Verification items for this drawing (mm, ordinates from the low corner). Round coordinates to 2 decimals unless told otherwise and drop trailing zeros. Order: outer loops, then holes, each group sorted by start corner. A loop starts at its lowest first (then second) coordinate and runs counter-clockwise, first axis right, second up. Notation, with made-up numbers: M -38.5,4.5 L -4.5,4.5 A20 cw -4.5,31.5 Z; hole C 1.25,85 d1. An arc over 180 degrees is marked long. One line per item, written item: value. Start each with the question number.
(1) Cross-section at A-A, the plane x = 3. Enter the section's corners in (y, z).
(2) Cross-section at C-C, the plane y = 1.1. Enter the section's corners in (x, z), and give its area (3 significant figures).
(3) Cross-section at D-D, the plane z = 9. Enter the section's corners in (x, y).
(4) Release check for a two-part mould opening along X. For the marked faces 1, 2 and 3 record: released by +X, released by -X, zero draft, split by the parting line, or undercut.
(5) Cross-section at B-B, the plane x = 11. Enter the section's corners in (y, z).
(6) Thickness scan on L1, parallel to Z at x = 3, y = 1.15; L2, parallel to X at y = 1, z = 7.5; L3, parallel to X at y = 0.65, z = 5.75. Record the ranges inside material, lowest first.
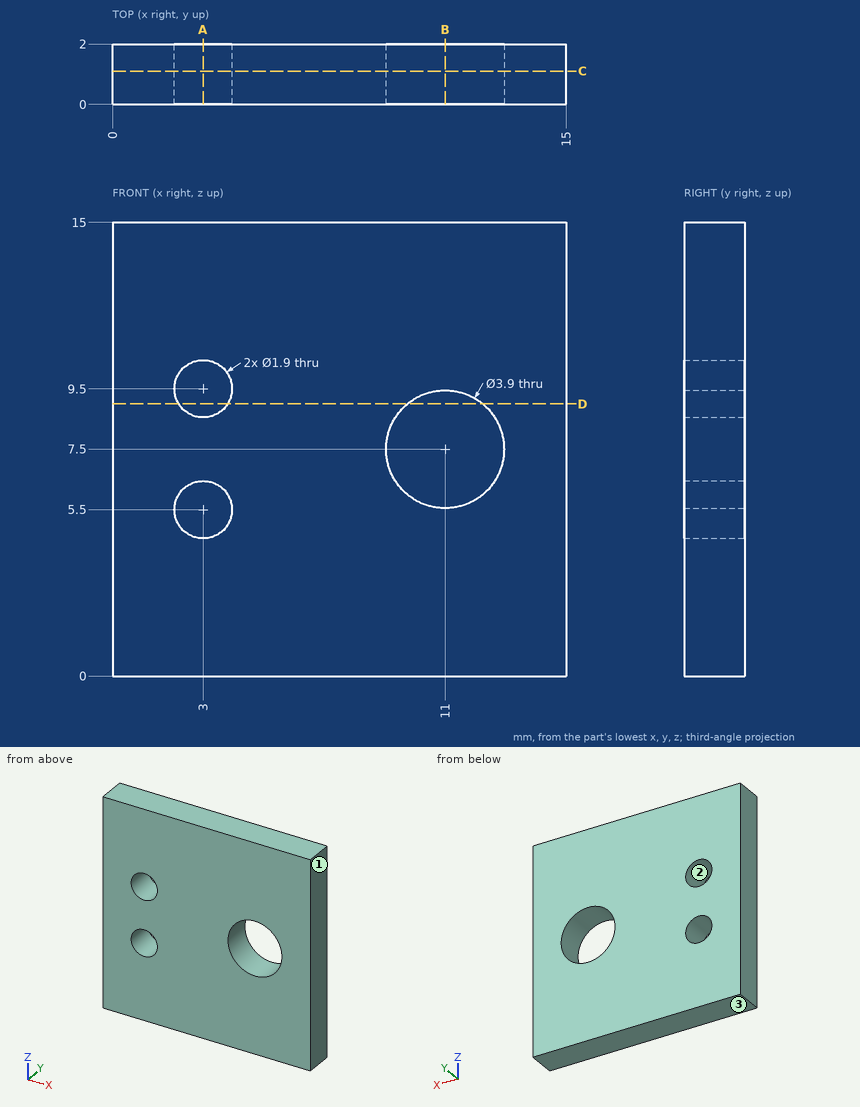
Values found:
1. outline: M 0,0 L 2,0 L 2,4.55 L 0,4.55 Z; M 0,6.45 L 2,6.45 L 2,8.55 L 0,8.55 Z; M 0,10.45 L 2,10.45 L 2,15 L 0,15 Z
2. outline: M 0,0 L 15,0 L 15,15 L 0,15 Z; hole C 3,5.5 d1.9; hole C 3,9.5 d1.9; hole C 11,7.5 d3.9
2. area: 207 mm^2
3. outline: M 0,0 L 2.19,0 L 2.19,2 L 0,2 Z; M 3.81,0 L 9.75,0 L 9.75,2 L 3.81,2 Z; M 12.25,0 L 15,0 L 15,2 L 12.25,2 Z
4. face 1: released by +X
4. face 2: undercut
4. face 3: zero draft
5. outline: M 0,0 L 2,0 L 2,5.55 L 0,5.55 Z; M 0,9.45 L 2,9.45 L 2,15 L 0,15 Z
6. L1: 0 to 4.55, 6.45 to 8.55, 10.45 to 15
6. L2: 0 to 9.05, 12.95 to 15
6. L3: 0 to 2.08, 3.92 to 10.14, 11.86 to 15
